from build123d import *

# Parameters (mm, degrees)
SKETCH_W     = 18
SKETCH_H     = 25.5
PAD_DEPTH    = 0.8
SKETCH001_R  = 0.25
POCKET_DEPTH = 5
PAD001_DEPTH = 0.1


with BuildPart() as part:
    # Sketch → Pad (new body)
    with BuildSketch(Plane.XY):
        with Locations((0, 12.75)):
            Rectangle(SKETCH_W, SKETCH_H)
    extrude(amount=-PAD_DEPTH)

    # Sketch001 → Pocket (cut)
    with BuildSketch(Plane.XY):
        with Locations((-5.715, 0)):
            Circle(SKETCH001_R)
        with Locations((-4.445, 0)):
            Circle(SKETCH001_R)
        with Locations((-3.175, 0)):
            Circle(SKETCH001_R)
        with Locations((-1.905, 0)):
            Circle(SKETCH001_R)
        with Locations((-0.635, 0)):
            Circle(SKETCH001_R)
        with Locations((0.635, 0)):
            Circle(SKETCH001_R)
        with Locations((1.905, 0)):
            Circle(SKETCH001_R)
        with Locations((3.175, 0)):
            Circle(SKETCH001_R)
        with Locations((4.445, 0)):
            Circle(SKETCH001_R)
        with Locations((5.715, 0)):
            Circle(SKETCH001_R)
        with Locations((-9, 1.5)):
            Circle(SKETCH001_R)
        with Locations((-9, 2.77)):
            Circle(SKETCH001_R)
        with Locations((-9, 4.04)):
            Circle(SKETCH001_R)
        with Locations((-9, 5.31)):
            Circle(SKETCH001_R)
        with Locations((-9, 6.58)):
            Circle(SKETCH001_R)
        with Locations((-9, 7.85)):
            Circle(SKETCH001_R)
        with Locations((-9, 9.12)):
            Circle(SKETCH001_R)
        with Locations((-9, 10.39)):
            Circle(SKETCH001_R)
        with Locations((-9, 11.66)):
            Circle(SKETCH001_R)
        with Locations((-9, 12.93)):
            Circle(SKETCH001_R)
        with Locations((-9, 14.2)):
            Circle(SKETCH001_R)
        with Locations((-9, 15.47)):
            Circle(SKETCH001_R)
        with Locations((-9, 16.74)):
            Circle(SKETCH001_R)
        with Locations((-9, 18.01)):
            Circle(SKETCH001_R)
        with Locations((9, 1.5)):
            Circle(SKETCH001_R)
        with Locations((9, 2.77)):
            Circle(SKETCH001_R)
        with Locations((9, 4.04)):
            Circle(SKETCH001_R)
        with Locations((9, 5.31)):
            Circle(SKETCH001_R)
        with Locations((9, 6.58)):
            Circle(SKETCH001_R)
        with Locations((9, 7.85)):
            Circle(SKETCH001_R)
        with Locations((9, 9.12)):
            Circle(SKETCH001_R)
        with Locations((9, 10.39)):
            Circle(SKETCH001_R)
        with Locations((9, 11.66)):
            Circle(SKETCH001_R)
        with Locations((9, 12.93)):
            Circle(SKETCH001_R)
        with Locations((9, 14.2)):
            Circle(SKETCH001_R)
        with Locations((9, 15.47)):
            Circle(SKETCH001_R)
        with Locations((9, 16.74)):
            Circle(SKETCH001_R)
        with Locations((9, 18.01)):
            Circle(SKETCH001_R)
    extrude(amount=-POCKET_DEPTH, mode=Mode.SUBTRACT)

    # Sketch002 → Pad001 (join)
    with BuildSketch(Plane.XY):
        Polygon((6.750327, 19.716486), (6.750327, 25.1), (1.77515, 25.1), (1.77515, 22.352757), (-0.253976, 22.352757), (-0.253976, 25.1), (-3.021827, 25.1), (-3.021827, 22.352757), (-5.009602, 22.352757), (-5.009602, 25.1), (-7.736101, 25.1), (-7.736101, 20.419491), (-7.236101, 20.419491), (-7.236101, 24.575495), (-5.509602, 24.575495), (-5.509602, 21.794554), (-2.521827, 21.794554), (-2.521827, 24.544479), (-0.753976, 24.544479), (-0.753976, 21.794554), (2.27515, 21.794554), (2.27515, 24.575495), (3.98755, 24.575495), (3.98755, 19.716486), (4.48755, 19.716486), (4.48755, 24.544479), (6.100327, 24.544479), (6.100327, 19.716486), align=None)
    extrude(amount=PAD001_DEPTH)


solid = part.part
Input: part model. Units: mm. Frame: model coordinates. Coordinates: 2 decimals unless noted, no trailing zeros. Write each loop counter-clockwise with the first axis right and the second up, starting at its lowest first coordinate (ties: lowest second). Pieces come first, ordered by that corner, then holes. Notation, with made-up numbers: M 22.25,41.5 L 67.25,41.5 A29 cw 67.25,66.5 Z; hole C 57.25,54 d6. An arc over 180 degrees is marked long. Answer as a JSON object with one key per item and string values. Group by question number.
(1) Contact query for a flat-ended pin moving along its axis: P1, Ø5, axis at x = -0.5, y = 17, coming from the +Z side. Output: stop coordinate, or through.
(2) Section B-B on x = 8.25. Output: boundary loops of the cut face in (y, z), plus the area to 3 significant figures.
(3) Section C-C on y = 13.5. Output: boundary loops of the cut face in (x, z).
(4) Mould query, pull axis X, two halves, no side actions, for faces 1 (the face through (0, 13, -0.8)), 2 (the face through (0, 13, 0)). Classes: pulls with the +X half, pulls with the -X half, needs draft (parallel to the pull), parting line crosses it, or undercut.
(5) Ray query, line 1 along Z through (x, y) = (-1, 20.75); line 2 along Y through (x, z) = (5.75, -0.55); line 3 along X through (y, z) = (18, -0.65). Return the intervals inside material, ascending. Write a range as [from, to].
Result set:
{
 "1": {"P1": "stops at z = 0"},
 "2": {"outline": "M 0,-0.8 L 25.5,-0.8 L 25.5,0 L 0,0 Z", "area": "20.4 mm2"},
 "3": {"outline": "M -9,-0.8 L 9,-0.8 L 9,0 L -9,0 Z"},
 "4": {"face 1": "needs draft", "face 2": "undercut"},
 "5": {"line 1": "z = [-0.8, 0]", "line 2": "y = [0.25, 25.5]", "line 3": "x = [-8.75, 8.75]"}
}
